CAD build for the part. Positions are in the model's coordinates, mm. A direction names the side the tool comes from. Give positions to 0.01 mm unless a question says otherwise; leave off trailing zeros. Loops run counter-clockwise (first coordinate to the right, second up) from the corner with the lowest first, then second, coordinate; pieces in that order, holes last. Notation, with made-up numbers: (39, 2.5) - (46, 2.5) arc R18 ccw to (46, 8.5) - close; hole circle Ø4 at (54.25, -23). An arc over 180 degrees is marked (long way). Return JSON: item names as keys, results as strings.
from build123d import *

# Parameters (mm, degrees)
SKETCH_1_W          = 2
SKETCH_1_H          = 12.1
EXTRUDE_1_DEPTH     = 13.2
SKETCH_2_W          = 0.330714911
SKETCH_2_H          = 1.671791026
CUT_EXTRUDE_1_DEPTH = 13.2


with BuildPart() as part:
    # 草图1 → 凸台-拉伸1 (new body)
    with BuildSketch(Plane(origin=(0, 0, 0), x_dir=(1, 0, 0), z_dir=(0, 1, 0))):
        Rectangle(SKETCH_1_W, SKETCH_1_H)
    extrude(amount=EXTRUDE_1_DEPTH)

    # 草图2 → 切除-拉伸1 (cut)
    with BuildSketch(Plane.ZY.offset(1)):
        with Locations((-5.884642545, 4.259492563)):
            Rectangle(SKETCH_2_W, SKETCH_2_H)
        Polygon((-4.518682009, 11.98), (-6.05, 9.129739953), (-6.05, 13.2), (6.05, 13.2), (6.05, 7.365579196), (3.461422835, 11.98), align=None)
    extrude(amount=-CUT_EXTRUDE_1_DEPTH, mode=Mode.SUBTRACT)


solid = part.part
1. Cut at B-B, the plane y = 4.25. Write the cut outline in (x, z), plus the area to 3 significant figures.
Values follow:
{"outline": "(-1, -5.72) - (1, -5.72) - (1, 6.05) - (-1, 6.05) - close", "area": "23.5 mm²"}
2. Cut at C-C, the plane z = 5. Write the cut outline in (x, y).
Values follow:
{"outline": "(-1, 0) - (1, 0) - (1, 9.24) - (-1, 9.24) - close"}
3. Cut at A-A, the plane x = -0.4. Write the cut outline in (y, z), plus the area to 3 significant figures.
Values follow:
{"outline": "(0, -6.05) - (3.42, -6.05) - (3.42, -5.72) - (5.1, -5.72) - (5.1, -6.05) - (9.13, -6.05) - (11.98, -4.52) - (11.98, 3.46) - (7.37, 6.05) - (0, 6.05) - close", "area": "136 mm²"}
4. Drill centre lines: probe 1 along Z at (x, y) = (-0.65, 3.5); probe 2 along Y at (x, z) = (0.05, 4); probe 3 along Y at (x, z) = (0.85, 3.5). Where is each one in solid material? Low to high.
Values follow:
{"probe 1": "z = -5.72 to 6.05", "probe 2": "y = 0 to 11.02", "probe 3": "y = 0 to 11.91"}
5. Which spindle directions (+Z, -Z, +X, -X, +Y, -Y) get a long thin tool onto all of the face, cutting with end or side? Do faces 1 (the face through (0, 11.98, 0)), 2 (the face through (0, 4, -5.719)). Say none if no direction does.
Values follow:
{"face 1": "+Z, -Z, +X, -X, +Y", "face 2": "-Z, +X, -X"}
6. Drop a flat-ended pin along its axis: P1, Ø0.8, axis at x = 0, y = 4.5, coming from the -Z side. Give the stop position or say it passes through.
Values follow:
{"P1": "stops at z = -5.72"}
